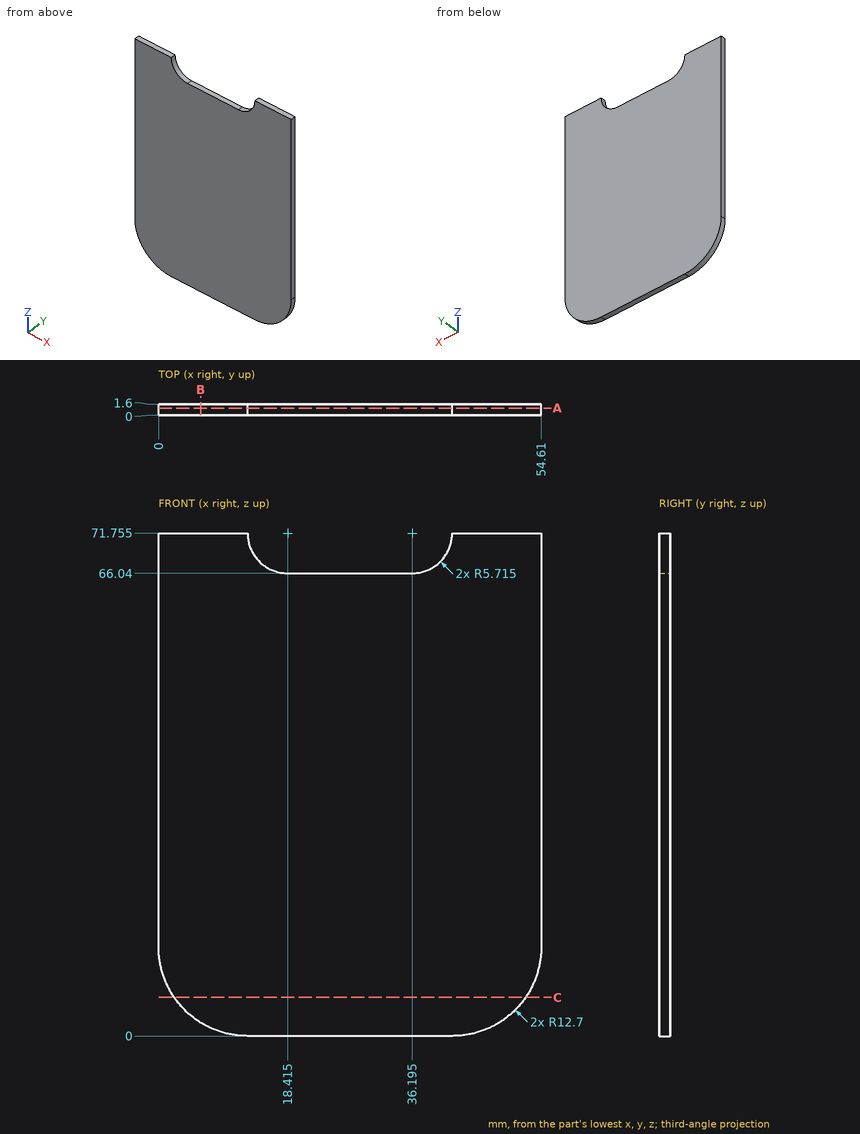
Design review of the part shown in the three views and the two pictorial views. Dimensions are in mm from the part's minimum x, y and z. Round coordinates to 2 decimals unless told otherwise and drop trailing zeros. Order: outer loops, then holes, each group sorted by start corner. A loop starts at its lowest first (then second) coordinate and runs counter-clockwise, first axis right, second up. Notation, with made-up numbers: (81.25, 40) -> (133.25, 40) arc R28 cw to (133.25, 61) -> close; hole circle Ø6 at (37.25, 86). An arc over 180 degrees is marked (long way). Write item = value, one per line. Start each with the question number.
1) Take a section at C-C on z = 5.5. State the section outline as (x, y) points.
2) Take a section at A-A on y = 1. State the section outline as (x, z) points (3 decimals).
3) To check wall thickness, follow line 1 (Z direction, x = 29.5, y = 1.45); line 2 (X direction, y = 1.5, z = 10.5); line 3 (Z direction, x = 16.5, y = 0.15). State the ranges of each line that lie inside material, in increasing order. Write a range as from..to.
4) Take a section at B-B on x = 6. State the section outline as (y, z) points (3 decimals).
Verdict:
q1.outline = (2.24, 0) -> (52.37, 0) -> (52.37, 1.6) -> (2.24, 1.6) -> close
q2.outline = (0, 12.7) arc R12.7 ccw to (12.7, 0) -> (41.91, 0) arc R12.7 ccw to (54.61, 12.7) -> (54.61, 71.755) -> (41.91, 71.755) arc R5.715 cw to (36.195, 66.04) -> (18.415, 66.04) arc R5.715 cw to (12.7, 71.755) -> (0, 71.755) -> close
q3.line_1 = 0..66.04
q3.line_2 = 0.19..54.42
q3.line_3 = 0..66.37
q4.outline = (0, 1.911) -> (1.6, 1.911) -> (1.6, 71.755) -> (0, 71.755) -> close
